from build123d import *

# Parameters (mm, degrees)
SKETCH_3_R          = 2.5
SKETCH_4_W          = 7.512886461
SKETCH_4_H          = 4
CUT_EXTRUDE_1_DEPTH = 10
CUT_EXTRUDE_START   = 10
SKETCH_4_3_W        = 9.374325773
SKETCH_4_3_H        = 4
CUT_EXTRUDE_2_DEPTH = 40.56056908
CUT_EXTRUDE_START_2 = -5
SKETCH_5_R          = 2.5
SKETCH_5_R_2        = 1.5
CUT_EXTRUDE_3_DEPTH = 5
CHAMFER_1_SIZE2     = 1
CHAMFER_1_SIZE      = 1.732050808


with BuildPart() as part:
    # 스윕1: sweep along a path in 스케치2
    with BuildLine(Plane.XY) as sweep_1_path:
        Line((7.5, -10), (7.5, 5))
        ThreePointArc((7.5, 5), (20, 17.5), (32.5, 5))
        Line((32.5, 5), (32.5, -35))
    # 스케치3 → 스윕1 (sweep)
    with BuildSketch(Plane(origin=(0, 0, 0), x_dir=(1, 0, 0), z_dir=(0, 1, 0))):
        with Locations((7.5, 0)):
            Circle(SKETCH_3_R)
    sweep(path=sweep_1_path.line)

    # 스케치4 → 컷-돌출1 (cut)
    with BuildSketch(Plane(origin=(0, 0, 0), x_dir=(0, 0, -1), z_dir=(1, 0, 0))):
        with Locations((5.256443231, -6)):
            Rectangle(SKETCH_4_W, SKETCH_4_H)
        Polygon((2.5, -10), (2.5, -8.5), (1.3, -10), align=None)
    extrude(amount=CUT_EXTRUDE_1_DEPTH, mode=Mode.SUBTRACT)

    # 스케치4<3> → 컷-돌출2 (cut, through all)
    with BuildSketch(Plane(origin=(0, 0, 0), x_dir=(0, 0, -1), z_dir=(1, 0, 0)).offset(CUT_EXTRUDE_START)):
        with Locations((-6.187162887, -6)):
            Rectangle(SKETCH_4_3_W, SKETCH_4_3_H)
        Polygon((-1.3, -35), (-2.5, -35), (-2.5, -33.5), align=None)
    extrude(amount=CUT_EXTRUDE_2_DEPTH, mode=Mode.SUBTRACT)

    # 스케치5 → 컷-돌출3 (cut)
    with BuildSketch(Plane.XZ.offset(35).offset(CUT_EXTRUDE_START_2)):
        with Locations((32.5, 0)):
            Circle(SKETCH_5_R)
        with Locations((32.5, 0)):
            Circle(SKETCH_5_R_2, mode=Mode.SUBTRACT)
    extrude(amount=-CUT_EXTRUDE_3_DEPTH, mode=Mode.SUBTRACT)

    # 모따기1
    chamfer_1_edges = [part.edges().sort_by_distance(p)[0] for p in [
        (35, -25, 0),
    ]]
    chamfer_1_side = [part.faces().sort_by_distance(p)[0] for p in [
        (35, -24.98, 0),
    ]]
    chamfer(chamfer_1_edges, length=CHAMFER_1_SIZE - 0.0001, length2=CHAMFER_1_SIZE2 - 0.0001, reference=chamfer_1_side[0])  # a hair under: the kernel refuses the full size


solid = part.part
Geometry check sheet. Reference: the model listing, model coordinates, mm. A direction names the side the tool comes from. Give positions to 0.01 mm unless a question says otherwise; leave off trailing zeros. Write each loop counter-clockwise with the first axis right and the second up, starting at its lowest first coordinate (ties: lowest second). Pieces come first, ordered by that corner, then holes.
1) Set-up check for faces 4 (the face through (34, -30, -1)), 5 (the face through (7.47, -9.406, -1.775)), 6 (the face through (32, -4, 2)), 7 (the face through (8, -10, 1)): record each of +Z, -Z, +X, -X, +Y, -Y from which the full face is reachable in a straight line by a thin tool's end or side.
Values follow:
face 4: none
face 5: -Z, -X, -Y
face 6: +Z, +X
face 7: +Z, -Z, -X, -Y
2) Cross-section at B-B (y = -31). Record the boundary of the cut face in (x, z), plus the area to 3 significant figures.
Values follow:
outline: circle Ø5 at (32.5, 0)
area: 19.6 mm2
3) Thickness scan on line 1 (X direction, y = -2.5, z = -1.5); line 2 (X direction, y = -4.5, z = -1.3); line 3 (X direction, y = -19.5, z = 0.1). Record the ranges inside material, lowest first.
Values follow:
line 1: x = 5.5 to 9.5, 30.5 to 34.5
line 2: x = 5.36 to 9.64, 30.36 to 34.64
line 3: x = 30 to 35
4) Go/stop test with flat-tipped pins: pin 1 Ø3 at (x, z) = (8, -0.5) entering from -Y; pin 2 Ø0.5 at (x, z) = (8, -2) entering from -Y; pin 3 Ø1.5 at (x, z) = (32.5, 0) entering from +Y. Record where each tip stops, or that it passes through.
Values follow:
pin 1: stops at y = -10
pin 2: stops at y = -9.44
pin 3: stops at y = 14.32
5) Release check for a two-part mould opening along X. For faces 1 (the face through (32.83, -32.53, -2.48)), 2 (the face through (7, -4, -2)), 3 (the face through (32.83, -9.33, -2.48)) record: released by +X, released by -X, zero draft, split by the parting line, or undercut.
Values follow:
face 1: split by the parting line
face 2: zero draft
face 3: undercut
